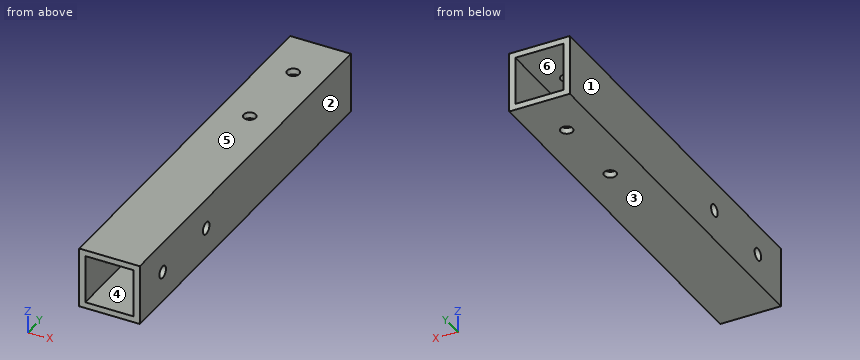
```python
from build123d import *

# Parameters (mm, degrees)
SKETCH_1_W              = 15
SKETCH_1_H              = 15
SKETCH_1_W_2            = 12
SKETCH_1_H_2            = 12
EXTRUDE_1_DEPTH         = 96.9
SKETCH_2_R              = 1.5
CUT_EXTRUDE_1_DEPTH     = 100.194808332
CUT_EXTRUDE_2_OUTLINE_R = 1.5
CUT_EXTRUDE_2_DEPTH     = 15


# Read off the part's stored shape, not the designer's step: 切除-拉伸2
with BuildPart() as part:
    # 草图1 → 凸台-拉伸1 (new body)
    with BuildSketch(Plane(origin=(0, 0, 0), x_dir=(1, 0, 0), z_dir=(0, 1, 0))):
        with Locations((7.5, 7.5)):
            Rectangle(SKETCH_1_W, SKETCH_1_H)
        with Locations((7.5, 7.5)):
            Rectangle(SKETCH_1_W_2, SKETCH_1_H_2, mode=Mode.SUBTRACT)
    extrude(amount=EXTRUDE_1_DEPTH)

    # 草图2 (on Front Plane) → 切除-拉伸1 (cut, through all)
    with BuildSketch(Plane.XY):
        with Locations((7.5, 64.4)):
            Circle(SKETCH_2_R)
        with Locations((7.5, 84.4)):
            Circle(SKETCH_2_R)
    extrude(amount=-CUT_EXTRUDE_1_DEPTH, mode=Mode.SUBTRACT)

    # 切除-拉伸2 outline → 切除-拉伸2 (cut)
    with BuildSketch(Plane.YZ):
        with Locations((10.5, -7.5)):
            Circle(CUT_EXTRUDE_2_OUTLINE_R)
        with Locations((30.5, -7.5)):
            Circle(CUT_EXTRUDE_2_OUTLINE_R)
    extrude(amount=CUT_EXTRUDE_2_DEPTH, mode=Mode.SUBTRACT)


solid = part.part
```
Geometry: final body of the model. Coordinates: model frame, mm. Face numbers are marked on the shaded views. A direction names the side the tool comes from. Round coordinates to 2 decimals unless told otherwise and drop trailing zeros. Order: outer loops, then holes, each group sorted by start corner. A loop starts at its lowest first (then second) coordinate and runs counter-clockwise, first axis right, second up. Notation, with made-up numbers: (65, -9.75) -> (105, -9.75) arc R31 ccw to (105, 14.25) -> close; hole circle Ø4 at (-10.75, 63). An arc over 180 degrees is marked (long way). Write each question's results on one line, items separated by ' | '.
Q1. Section query B-B (y = 64.4). Output: boundary loops of the cut face in (x, z).
Response values:
outline: (0, -15) -> (6, -15) -> (6, -13.5) -> (1.5, -13.5) -> (1.5, -1.5) -> (6, -1.5) -> (6, 0) -> (0, 0) -> close; (9, -15) -> (15, -15) -> (15, 0) -> (9, 0) -> (9, -1.5) -> (13.5, -1.5) -> (13.5, -13.5) -> (9, -13.5) -> close
Q2. Section query A-A (z = -10.5). Output: boundary loops of the cut face in (x, y), and give its area (3 significant figures).
Response values:
outline: (0, 0) -> (1.5, 0) -> (1.5, 96.9) -> (0, 96.9) -> close; (13.5, 0) -> (15, 0) -> (15, 96.9) -> (13.5, 96.9) -> close | area: 291 mm²
Q3. Section query C-C (y = 21). Output: boundary loops of the cut face in (x, z), and give its area (3 significant figures).
Response values:
outline: (0, -15) -> (15, -15) -> (15, 0) -> (0, 0) -> close; hole (1.5, -13.5) -> (13.5, -13.5) -> (13.5, -1.5) -> (1.5, -1.5) -> close | area: 81.0 mm²
Q4. Pull-direction query (X, two-part tool) for the marked faces 1, 2, 3 and 4; classes: released by +X, released by -X, zero draft, split by the parting line, or undercut.
Response values:
face 1: released by -X | face 2: released by +X | face 3: zero draft | face 4: undercut
Q5. Section query D-D (x = 7.5). Output: boundary loops of the cut face in (y, z), and give its area (3 significant figures).
Response values:
outline: (0, -15) -> (62.9, -15) -> (62.9, -13.5) -> (0, -13.5) -> close; (0, -1.5) -> (62.9, -1.5) -> (62.9, 0) -> (0, 0) -> close; (65.9, -15) -> (82.9, -15) -> (82.9, -13.5) -> (65.9, -13.5) -> close; (65.9, -1.5) -> (82.9, -1.5) -> (82.9, 0) -> (65.9, 0) -> close; (85.9, -15) -> (96.9, -15) -> (96.9, -13.5) -> (85.9, -13.5) -> close; (85.9, -1.5) -> (96.9, -1.5) -> (96.9, 0) -> (85.9, 0) -> close | area: 273 mm²
Q6. Ray query, line 1 along Y through (x, z) = (7.5, -0.85); line 2 along Y through (x, z) = (14.75, -7.5); line 3 along Z through (x, y) = (5.75, 57). Return the intervals inside material, ascending.
Response values:
line 1: 0 to 62.9, 65.9 to 82.9, 85.9 to 96.9 | line 2: 0 to 9, 12 to 29, 32 to 96.9 | line 3: -15 to -13.5, -1.5 to 0
Q7. Access query for the marked faces 5 and 6. Directions: +Z, -Z, +X, -X, +Y, -Y. A direction counts if a zero-diameter tool reaches every point of the face in a straight line with its end or side. Return the directions, or none.
Response values:
face 5: +Z, +X, -X, +Y, -Y | face 6: +Y, -Y
